Source: CAD feature listing. Evaluate the final solid. Frame: model axes, mm. A direction names the side the tool comes from. Give positions to 0.01 mm unless a question says otherwise; leave off trailing zeros. Use one line per item in the form item = value. Start each with the question number.
(1) Cut plane A-A, the plane z = 27. Count the separate pieces of the cut face and the enclosed holes in it, and give its area (3 significant figures).
(2) Draft query along Z for faces 3 (the face through (-57, 85.115, -10)), 4 (the face through (0.83, -48.77, 15.36)), 5 (the face through (29.348, 62.068, -56.426)). Return one class per face: pulls with the +Z half, pulls with the -Z half, needs draft (parallel to the pull), parting line crosses it, or undercut.
(3) Set-up query: faces 1 (the face through (85.115, 10, 57)), 2 (the face through (-37.685, 42.183, -34.556)). Return all of +Z, -Z, +X, -X, +Y, -Y with unobstructed straight access to the full face (end or side cutting, diameter ignored); none if empty.
(4) Material intervals for line 1 along Z through (x, y) = (-51, -0.5); line 2 along X through (y, z) = (55, 7); line 3 along Z through (x, y) = (-55, 14), sorted ascending. Write a range as from..to.
(5) First-contact query: P1, Ø6, axis at x = 29.5, z = -24.5, coming from the +Y side; P2, Ø12, axis at x = -36.5, y = 21.5, coming from the +Z side; P3, Ø8, axis at x = -38, z = 4, coming from the -Y side; P4, Ø6, axis at y = 51, z = 3.5, coming from the +X side. Flat tips, straight axial feed; report the tip coordinate or a pass-through.
from build123d import *

# Parameters (mm, degrees)
SKETCH4_R           = 63.6016
BOSS_EXTRUDE1_DEPTH = 117.9576
SKETCH5_R           = 63.6016
BOSS_EXTRUDE2_DEPTH = 58.9788
SKETCH8_R           = 63.6016
SKETCH8_R_2         = 47.397505823
CUT_EXTRUDE1_DEPTH  = 25.4
SKETCH9_R           = 79.726534617
SKETCH9_R_2         = 24.880704632
CUT_EXTRUDE2_DEPTH  = 25.4
SKETCH10_R          = 82.836499496
SKETCH10_R_2        = 21.967276082
CUT_EXTRUDE3_DEPTH  = 25.4


with BuildPart() as part:
    # Sketch1 → Revolve1 (revolve)
    with BuildSketch(Plane.XY):
        Polygon((-110.5154, -63.6016), (-58.9788, -63.6016), (-58.9788, -57.0357), (-110.5154, -57.3786), align=None)
        Polygon((110.5154, -57.3786), (58.9788, -57.0357), (58.9788, -63.6016), (110.5154, -63.6016), align=None)
    revolve(axis=Axis((-110.5154, 0, 0), (1, 0, 0)))



with BuildPart() as body_2:
    # Sketch2 → Revolve2 (revolve)
    with BuildSketch(Plane.XY):
        Polygon((57.3786, 110.5154), (57.0357, 58.9788), (63.6016, 58.9788), (63.6016, 110.5154), align=None)
    revolve(axis=Axis((0, 0, 0), (0, 1, 0)))


with BuildPart() as part_1:
    add(part.part)

    add(body_2.part)  # Boss-Extrude1 merges body 2
    # Sketch4 → Boss-Extrude1 (add)
    with BuildSketch(Plane(origin=(-58.9788, 0, 0), x_dir=(0, 0, -1), z_dir=(1, 0, 0))):
        Circle(SKETCH4_R)
    extrude(amount=BOSS_EXTRUDE1_DEPTH)

    # Sketch5 → Boss-Extrude2 (add)
    with BuildSketch(Plane.XZ.offset(-58.9788)):
        Circle(SKETCH5_R)
    extrude(amount=BOSS_EXTRUDE2_DEPTH)

    # Sketch6 → Cut-Revolve1 (revolve, cut)
    with BuildSketch(Plane.XY):
        Polygon((-110.5154, -57.3786), (-58.9788, -57.0357), (-58.9788, -51.1302), (58.9788, -51.1302), (58.9788, -57.0357), (110.5154, -57.3786), (110.5154, 0), (-110.5154, 0), align=None)
    revolve(axis=Axis((110.5154, 0, 0), (-1, 0, 0)), mode=Mode.SUBTRACT)

    # Sketch7 → Cut-Revolve2 (revolve, cut)
    with BuildSketch(Plane.XY):
        Polygon((57.3786, 110.5154), (57.0357, 58.9788), (51.1302, 58.9788), (51.1302, 0), (0, 0), (0, 110.5154), align=None)
    revolve(axis=Axis((0, 0, 0), (0, 1, 0)), mode=Mode.SUBTRACT)

    # Sketch8 → Cut-Extrude1 (cut)
    with BuildSketch(Plane(origin=(0, 110.5154, 0), x_dir=(1, 0, 0), z_dir=(0, 1, 0))):
        Circle(SKETCH8_R)
        Circle(SKETCH8_R_2, mode=Mode.SUBTRACT)
    extrude(amount=-CUT_EXTRUDE1_DEPTH, mode=Mode.SUBTRACT)

    # Sketch9 → Cut-Extrude2 (cut)
    with BuildSketch(Plane.ZY.offset(110.5154)):
        Circle(SKETCH9_R)
        Circle(SKETCH9_R_2, mode=Mode.SUBTRACT)
    extrude(amount=-CUT_EXTRUDE2_DEPTH, mode=Mode.SUBTRACT)

    # Sketch10 → Cut-Extrude3 (cut)
    with BuildSketch(Plane(origin=(110.5154, 0, 0), x_dir=(0, 0, -1), z_dir=(1, 0, 0))):
        Circle(SKETCH10_R)
        Circle(SKETCH10_R_2, mode=Mode.SUBTRACT)
    extrude(amount=-CUT_EXTRUDE3_DEPTH, mode=Mode.SUBTRACT)


solid = part_1.part
Geometry says:
q1.separate_pieces = 3
q1.enclosed_holes = 0
q1.area = 3,290 mm^2
q2.face_3 = needs draft
q2.face_4 = undercut
q2.face_5 = parting line crosses it
q3.face_1 = +Z, -Z, +X, +Y, -Y
q3.face_2 = +Y
q4.line_1 = -63.6..-51.13, 51.13..63.6
q4.line_2 = -58.98..-50.65, 50.65..58.98
q4.line_3 = -62.04..-49.18, 49.18..62.04
q5.P1 = -43.11
q5.P2 = 61.68
q5.P3 = -63.6
q5.P4 = 58.98
